```python
from build123d import *

# Parameters (mm, degrees)
SKETCH_1_W               = 300
SKETCH_1_H               = 300
EXTRUDE_1_DEPTH          = 7
SKETCH_2_W               = 240
SKETCH_2_H               = 2.5
CUT_EXTRUDE_1_DEPTH      = 50
SKETCH_3_W               = 60
SKETCH_3_H               = 2.5
CUT_EXTRUDE_2_DEPTH      = 50
CUT_EXTRUDE_3_DEPTH      = 50
CUT_EXTRUDE_4_DEPTH      = 50
CUT_EXTRUDE_5_DEPTH      = 50
SKETCH_7_W               = 35
SKETCH_7_H               = 60
CUT_EXTRUDE_6_DEPTH      = 50
SKETCH_8_R               = 1.5
CUT_EXTRUDE_7_DEPTH      = 500
FILLET_1_R               = 10
FILLET_2_R               = 10
FILLET_3_R               = 10
FILLET_4_R               = 10
FILLET_5_R               = 10
FILLET_6_R               = 10
SKETCH_9_R               = 1.5
CUT_EXTRUDE_8_DEPTH      = 50
PATTERN_CIRCULAR_1_COUNT = 10
SKETCH_11_R              = 3.300758287
SKETCH_11_R_2            = 5.737524446
SKETCH_11_R_3            = 4.850679924
SKETCH_11_R_4            = 5.043067488
EXTRUDE_3_DEPTH          = 7
CUT_EXTRUDE_9_DEPTH      = 50
SKETCH_14_R              = 1.5
CUT_EXTRUDE_10_DEPTH     = 50
SKETCH_15_R              = 1.5
CUT_EXTRUDE_11_DEPTH     = 50


with BuildPart() as part:
    # 草图1 → 凸台-拉伸1 (new body)
    with BuildSketch(Plane(origin=(0, 0, 0), x_dir=(1, 0, 0), z_dir=(0, 1, 0))):
        Rectangle(SKETCH_1_W, SKETCH_1_H)
    extrude(amount=EXTRUDE_1_DEPTH)

    # 草图2 → 切除-拉伸1 (cut)
    with BuildSketch(Plane(origin=(0, 7, 0), x_dir=(1, 0, 0), z_dir=(0, 1, 0))):
        with Locations((-30, -148.75)):
            Rectangle(SKETCH_2_W, SKETCH_2_H)
    extrude(amount=-CUT_EXTRUDE_1_DEPTH, mode=Mode.SUBTRACT)

    # 草图3 → 切除-拉伸2 (cut)
    with BuildSketch(Plane(origin=(0, 7, 0), x_dir=(1, 0, 0), z_dir=(0, 1, 0))):
        with Locations((120, -148.75)):
            Rectangle(SKETCH_3_W, SKETCH_3_H)
    extrude(amount=-CUT_EXTRUDE_2_DEPTH, mode=Mode.SUBTRACT)

    # 草图4 → 切除-拉伸3 (cut)
    with BuildSketch(Plane(origin=(0, 7, 0), x_dir=(1, 0, 0), z_dir=(0, 1, 0))):
        Polygon((-60.234749658, 147.5), (-150, 147.5), (-150, 150), (150, 150), (150, 148.75), (150, 147.5), align=None)
    extrude(amount=-CUT_EXTRUDE_3_DEPTH, mode=Mode.SUBTRACT)

    # 草图5 → 切除-拉伸4 (cut)
    with BuildSketch(Plane(origin=(0, 7, 0), x_dir=(1, 0, 0), z_dir=(0, 1, 0))):
        Polygon((-145, -36.273195626), (-145, -168.077464091), (-167.085104341, -168.077464091), (-167.085104341, 166.966608586), (-145, 166.966608586), align=None)
    extrude(amount=-CUT_EXTRUDE_4_DEPTH, mode=Mode.SUBTRACT)

    # 草图6 → 切除-拉伸5 (cut)
    with BuildSketch(Plane(origin=(0, 7, 0), x_dir=(1, 0, 0), z_dir=(0, 1, 0))):
        Polygon((150, -147.5), (150, 173.372620909), (145, 173.372620909), (145, -12.70619331), (145, -195.232190074), (157.067783109, -195.232190074), align=None)
    extrude(amount=-CUT_EXTRUDE_5_DEPTH, mode=Mode.SUBTRACT)

    # 草图7 → 切除-拉伸6 (cut)
    with BuildSketch(Plane.XZ):
        with Locations((-127.5, 117.5)):
            Rectangle(SKETCH_7_W, SKETCH_7_H)
        with Locations((-127.5, -117.5)):
            Rectangle(SKETCH_7_W, SKETCH_7_H)
        with Locations((127.5, 117.5)):
            Rectangle(SKETCH_7_W, SKETCH_7_H)
        with Locations((127.5, -117.5)):
            Rectangle(SKETCH_7_W, SKETCH_7_H)
    extrude(amount=-CUT_EXTRUDE_6_DEPTH, mode=Mode.SUBTRACT)

    # 草图8 → 切除-拉伸7 (cut)
    with BuildSketch(Plane(origin=(0, 7, 0), x_dir=(1, 0, 0), z_dir=(0, 1, 0))):
        with Locations(Location((-125, 50, 0), (0, 0, 270))):
            Circle(SKETCH_8_R)
        with Locations(Location((-125, -50, 0), (0, 0, 270))):
            Circle(SKETCH_8_R)
        with Locations(Location((125, -50, 0), (0, 0, 270))):
            Circle(SKETCH_8_R)
        with Locations(Location((125, 50, 0), (0, 0, 270))):
            Circle(SKETCH_8_R)
        with Locations(Location((-80, 70, 0), (0, 0, 270))):
            Circle(SKETCH_8_R)
        with Locations(Location((80, 70, 0), (0, 0, 270))):
            Circle(SKETCH_8_R)
        with Locations(Location((0, 70, 0), (0, 0, 270))):
            Circle(SKETCH_8_R)
        with Locations(Location((0, -132.5, 0), (0, 0, 270))):
            Circle(SKETCH_8_R)
        with Locations(Location((-85, -82.5, 0), (0, 0, 270))):
            Circle(SKETCH_8_R)
        with Locations(Location((85, -82.5, 0), (0, 0, 270))):
            Circle(SKETCH_8_R)
    extrude(amount=-CUT_EXTRUDE_7_DEPTH, mode=Mode.SUBTRACT)

    # 圆角1
    fillet_1_edges = [part.edges().sort_by_distance(p)[0] for p in [
        (110, 3.5, 147.5),
        (-110, 3.5, 147.5),
    ]]
    fillet(fillet_1_edges, radius=FILLET_1_R)

    # 圆角2
    fillet_2_edges = [part.edges().sort_by_distance(p)[0] for p in [
        (110, 3.5, 87.5),
        (-110, 3.5, 87.5),
    ]]
    fillet(fillet_2_edges, radius=FILLET_2_R)

    # 圆角3
    fillet_3_edges = [part.edges().sort_by_distance(p)[0] for p in [
        (145, 3.5, 87.5),
        (-145, 3.5, 87.5),
    ]]
    fillet(fillet_3_edges, radius=FILLET_3_R)

    # 圆角4
    fillet_4_edges = [part.edges().sort_by_distance(p)[0] for p in [
        (145, 3.5, -87.5),
        (-145, 3.5, -87.5),
    ]]
    fillet(fillet_4_edges, radius=FILLET_4_R)

    # 圆角5
    fillet_5_edges = [part.edges().sort_by_distance(p)[0] for p in [
        (-110, 3.5, -87.5),
        (110, 3.5, -87.5),
    ]]
    fillet(fillet_5_edges, radius=FILLET_5_R)

    # 圆角6
    fillet_6_edges = [part.edges().sort_by_distance(p)[0] for p in [
        (-110, 3.5, -147.5),
        (110, 3.5, -147.5),
    ]]
    fillet(fillet_6_edges, radius=FILLET_6_R)

    # 草图9 → 切除-拉伸8 (cut)
    with BuildSketch(Plane(origin=(0, 7, 0), x_dir=(1, 0, 0), z_dir=(0, 1, 0))):
        with Locations(Location((0, 125, 0), (0, 0, 270))):
            Circle(SKETCH_9_R)
    cut_extrude_8 = extrude(amount=-CUT_EXTRUDE_8_DEPTH, mode=Mode.SUBTRACT)

    # 阵列(圆周)1: 切除-拉伸8 ×10 about axis
    pattern_circular_1_axis = Axis((0, 0, -70), (0, 1, 0))
    for i in range(1, PATTERN_CIRCULAR_1_COUNT):
        add(cut_extrude_8.rotate(pattern_circular_1_axis, i * 360 / PATTERN_CIRCULAR_1_COUNT), mode=Mode.SUBTRACT)

    # 草图11 → 凸台-拉伸3 (add)
    with BuildSketch(Plane(origin=(0, 7, 0), x_dir=(1, 0, 0), z_dir=(0, 1, 0))):
        with Locations((-32.328188876, 114.495934691)):
            Circle(SKETCH_11_R)
        with Locations((32.328188876, 114.495934691)):
            Circle(SKETCH_11_R_2)
        with Locations((-32.328188876, 25.504065309)):
            Circle(SKETCH_11_R_3)
        with Locations((32.328188876, 25.504065309)):
            Circle(SKETCH_11_R_4)
    extrude(amount=-EXTRUDE_3_DEPTH)

    # 草图12 → 切除-拉伸9 (cut)
    with BuildSketch(Plane.XZ):
        with BuildLine():
            Line((-20, 17.5), (20, 17.5))
            ThreePointArc((20, 17.5), (30, 7.5), (20, -2.5))
            Line((20, -2.5), (-20, -2.5))
            ThreePointArc((-20, -2.5), (-30, 7.5), (-20, 17.5))
        make_face()
    extrude(amount=-CUT_EXTRUDE_9_DEPTH, mode=Mode.SUBTRACT)

    # 草图14 → 切除-拉伸10 (cut)
    with BuildSketch(Plane.XZ):
        with Locations((0, 132)):
            Circle(SKETCH_14_R)
        with Locations(Location((-50, 82, 0), (0, 0, 270))):
            Circle(SKETCH_14_R)
        with Locations(Location((50, 82, 0), (0, 0, 270))):
            Circle(SKETCH_14_R)
        with Locations(Location((0, 32, 0), (0, 0, 270))):
            Circle(SKETCH_14_R)
    extrude(amount=-CUT_EXTRUDE_10_DEPTH, mode=Mode.SUBTRACT)

    # 草图15 → 切除-拉伸11 (cut)
    with BuildSketch(Plane.XZ):
        with Locations(Location((0, 117.5, 0), (0, 0, 270))):
            Circle(SKETCH_15_R)
    extrude(amount=-CUT_EXTRUDE_11_DEPTH, mode=Mode.SUBTRACT)


solid = part.part
```
Here's how the part is built. I have some questions about the finished solid (model axes, mm). A direction names the side the tool comes from. Coordinates: 2 decimals unless noted, no trailing zeros. Order: outer loops, then holes, each group sorted by start corner. A loop starts at its lowest first (then second) coordinate and runs counter-clockwise, first axis right, second up.
1) Will these pins go through, and if not, where does the flat tip stop? pin 1 (3 mm diameter, centred on y = 4, z = -108, fed in from +X); pin 2 (1.8 mm diameter, centred on x = 52.31, z = -53, fed in from -Y); pin 3 (2 mm diameter, centred on y = 4, z = -85, fed in from +X).
2) Imagine slicing it at C-C on y = 5.5. State how many separate pieces and enclosed holes the cut face has, and give its area (3 significant figures).
3) We'd pull the mould along X, two halves only. Please class faces 5 (the face through (112.85, 3.55, 90.51)), 6 (the face through (30, 0, -2)), 7 (the face through (-30, 3.5, 7.3)): +X half, -X half, draft (parallel to the pull), parting line (faces both ways), or undercut.
4) Imagine slicing it at B-B on z = 5. List the corners of the cut face in (x, y) for me, and give its area (3 significant figures).
5) Which directions (+Z, -Z, +X, -X, +Y, -Y) give clear straight access to the entire face, cutting with the end or side of a thin tool? Please do faces 1 (the face through (110, 3, 117)), 2 (the face through (-110, 3, 117)), 3 (the face through (110, 3, -118)), 4 (the face through (0, 3, -2.5)).
6) I need wall thicknesses on line 1 (Z direction, x = 20, y = 6.75); line 2 (X direction, y = 2, z = 132); line 3 (X direction, y = 3.75, z = 32). Which ranges of each line are inside material? Lowest first, please.
7) Imagine slicing it at A-A on x = -11. List the corners of the cut face in (y, z) for me, and give its area (4 significant figures).
Response values:
1. pin 1: stops at x = 110
1. pin 2: passes through
1. pin 3: stops at x = 142.6
2. separate pieces: 1
2. enclosed holes: 21
2. area: 75,800 mm2
3. face 5: +X half
3. face 6: draft
3. face 7: undercut
4. outline: (-145, 0) - (-29.68, 0) - (-29.68, 7) - (-145, 7) - close; (29.68, 0) - (145, 0) - (145, 7) - (29.68, 7) - close
4. area: 1,610 mm2
5. face 1: +Z, +X, +Y, -Y
5. face 2: +Z, -X, +Y, -Y
5. face 3: -Z, +X, +Y, -Y
5. face 4: +Y, -Y
6. line 1: z = -147.5 to -2.5, 17.5 to 147.5
6. line 2: x = -110 to -1.5, 1.5 to 110
6. line 3: x = -145 to -1.5, 1.5 to 145
7. outline: (0, -147.5) - (7, -147.5) - (7, -2.5) - (0, -2.5) - close; (0, 17.5) - (7, 17.5) - (7, 147.5) - (0, 147.5) - close
7. area: 1,925 mm2
